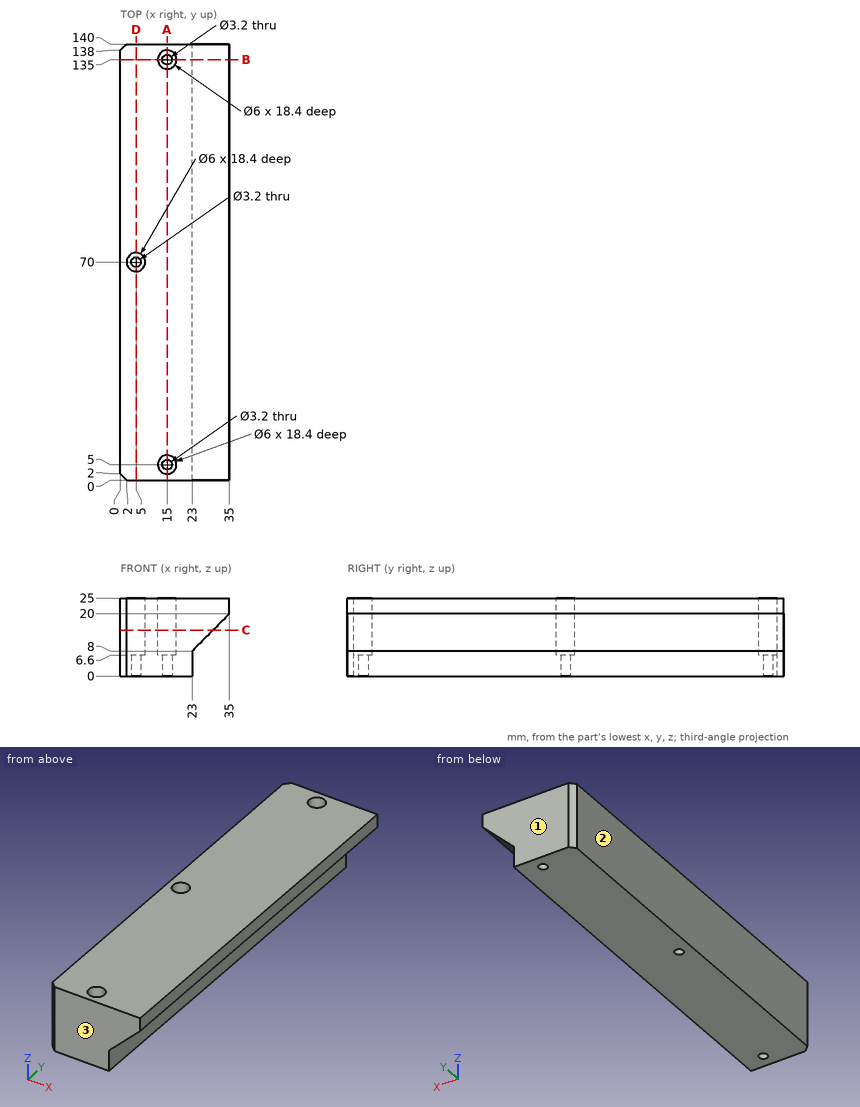
Part print with two shaded views. Sizes in mm from the minimum x, y, z corner. Give positions to 0.01 mm unless a question says otherwise; leave off trailing zeros. Order: outer loops, then holes, each group sorted by start corner. A loop starts at its lowest first (then second) coordinate and runs counter-clockwise, first axis right, second up.
(1) Drill centre lines: L1, parallel to Y at x = 15, z = 15.25; L2, parallel to Y at x = 15, z = 3.5; L3, parallel to X at y = 135, z = 20.5. Where is each one in solid material? Low to high.
(2) Saw through at D-D, the plane x = 5. Give the cut face in (y, z).
(3) Mould opens along Y. For the marked faces 1, 2 and 3 say: released by +Y, released by -Y, zero draft, split by the parting line, or undercut.
(4) Saw through at B-B, the plane y = 135. Give the cut face in (x, z), then the cut area to 3 significant figures.
(5) Flat gauge pins, fed straight in: pin 1 (1.8 mm diameter, centred on x = 6, y = 71.5, fed in from +Z); pin 2 (4 mm diameter, centred on y = 104, z = 5, fed in from +X); pin 3 (5 mm diameter, centred on y = 56, z = 6.5, fed in from +X). Where does each tip first touch, or does it go through?
(6) Saw through at C-C, the plane z = 14.75. Give the cut face in (x, y), then the cut area to 3 significant figures.
(7) Saw through at A-A, the plane x = 15. Give the cut face in (y, z), then the cut area to 3 significant figures.
Results found:
1. L1: y = 0 to 2, 8 to 132, 138 to 140
1. L2: y = 0 to 3.4, 6.6 to 133.4, 136.6 to 140
1. L3: x = 0 to 12, 18 to 35
2. outline: (0, 0) - (68.4, 0) - (68.4, 6.6) - (67, 6.6) - (67, 25) - (0, 25) - close; (71.6, 0) - (140, 0) - (140, 25) - (73, 25) - (73, 6.6) - (71.6, 6.6) - close
3. face 1: released by +Y
3. face 2: zero draft
3. face 3: released by -Y
4. outline: (0, 0) - (13.4, 0) - (13.4, 6.6) - (12, 6.6) - (12, 25) - (0, 25) - close; (16.6, 0) - (23, 0) - (23, 8) - (35, 20) - (35, 25) - (18, 25) - (18, 6.6) - (16.6, 6.6) - close
4. area: 575 mm2
5. pin 1: stops at z = 6.6
5. pin 2: stops at x = 23
5. pin 3: stops at x = 24
6. outline: (0, 2) - (2, 0) - (29.75, 0) - (29.75, 140) - (2, 140) - (0, 138) - close; hole circle Ø6 at (5, 70); hole circle Ø6 at (15, 5); hole circle Ø6 at (15, 135)
6. area: 4,080 mm2
7. outline: (0, 0) - (3.4, 0) - (3.4, 6.6) - (2, 6.6) - (2, 25) - (0, 25) - close; (6.6, 0) - (133.4, 0) - (133.4, 6.6) - (132, 6.6) - (132, 25) - (8, 25) - (8, 6.6) - (6.6, 6.6) - close; (136.6, 0) - (140, 0) - (140, 25) - (138, 25) - (138, 6.6) - (136.6, 6.6) - close
7. area: 3,240 mm2
